```python
from build123d import *

# Parameters (mm, degrees)
SKETCH_1_W          = 92
SKETCH_1_H          = 30
SKETCH_1_R          = 1.05
EXTRUDE_1_DEPTH     = 4
SKETCH_4_W          = 92
SKETCH_4_H          = 30
EXTRUDE_4_DEPTH     = 4
SKETCH_5_W          = 92
SKETCH_5_H          = 34
SKETCH_5_R          = 1.05
EXTRUDE_5_DEPTH     = 4
FILLET_4_R          = 2
CUT_EXTRUDE_1_DEPTH = 45
SKETCH_8_R          = 2.55
CUT_EXTRUDE_2_DEPTH = 5
SKETCH_9_W          = 7
SKETCH_9_H          = 21
SKETCH_9_R          = 1.05
EXTRUDE_6_DEPTH     = 6


with BuildPart() as part:
    # 草图1 → 凸台-拉伸1 (new body)
    with BuildSketch(Plane.XY):
        with Locations((46, -15)):
            Rectangle(SKETCH_1_W, SKETCH_1_H)
        with Locations((3.5, -5)):
            Circle(SKETCH_1_R, mode=Mode.SUBTRACT)
        with Locations((3.5, -20)):
            Circle(SKETCH_1_R, mode=Mode.SUBTRACT)
        with Locations((88.5, -5)):
            Circle(SKETCH_1_R, mode=Mode.SUBTRACT)
        with Locations((88.5, -20)):
            Circle(SKETCH_1_R, mode=Mode.SUBTRACT)
        with BuildLine():
            Line((43.45, -17.5), (43.45, -7.5))
            ThreePointArc((43.45, -7.5), (46, -4.95), (48.55, -7.5))
            Line((48.55, -7.5), (48.55, -17.5))
            ThreePointArc((48.55, -17.5), (46, -20.05), (43.45, -17.5))
        make_face(mode=Mode.SUBTRACT)
    extrude(amount=EXTRUDE_1_DEPTH)

    # 草图4 → 凸台-拉伸4 (add)
    with BuildSketch(Plane(origin=(0, -30, 0), x_dir=(-1, 0, 0), z_dir=(0, -1, 0))):
        with Locations((-46, -15)):
            Rectangle(SKETCH_4_W, SKETCH_4_H)
    extrude(amount=EXTRUDE_4_DEPTH)

    # 草图5 → 凸台-拉伸5 (add)
    with BuildSketch(Plane.XY.offset(30)):
        with Locations((46, -17)):
            Rectangle(SKETCH_5_W, SKETCH_5_H)
        with Locations((3.5, -5)):
            Circle(SKETCH_5_R, mode=Mode.SUBTRACT)
        with Locations((3.5, -20)):
            Circle(SKETCH_5_R, mode=Mode.SUBTRACT)
        with Locations((88.5, -20)):
            Circle(SKETCH_5_R, mode=Mode.SUBTRACT)
        with Locations((88.5, -5)):
            Circle(SKETCH_5_R, mode=Mode.SUBTRACT)
    extrude(amount=EXTRUDE_5_DEPTH)

    # 圆角4
    fillet_4_edges = [part.edges().sort_by_distance(p)[0] for p in [
        (46, -30, 30),
        (46, -34, 0),
        (46, -34, 34),
        (0, 0, 32),
        (92, 0, 32),
        (0, 0, 2),
        (92, 0, 2),
        (46, -30, 4),
    ]]
    fillet(fillet_4_edges, radius=FILLET_4_R)

    # 草图7 → 切除-拉伸1 (cut)
    with BuildSketch(Plane(origin=(0, 0, 0), x_dir=(-1, 0, 0), z_dir=(0, 0, -1))):
        with BuildLine():
            Line((-48.55, -17.5), (-48.55, -7.5))
            ThreePointArc((-48.55, -7.5), (-46, -4.95), (-43.45, -7.5))
            Line((-43.45, -7.5), (-43.45, -17.5))
            ThreePointArc((-43.45, -17.5), (-46, -20.05), (-48.55, -17.5))
        make_face()
    extrude(amount=-CUT_EXTRUDE_1_DEPTH, mode=Mode.SUBTRACT)

    # 草图8 → 切除-拉伸2 (cut)
    with BuildSketch(Plane(origin=(0, -34, 0), x_dir=(-1, 0, 0), z_dir=(0, -1, 0))):
        with Locations(Location((-46, -16.5, 0), (0, 0, 90))):
            Circle(SKETCH_8_R)
    extrude(amount=-CUT_EXTRUDE_2_DEPTH, mode=Mode.SUBTRACT)

    # 草图9 → 凸台-拉伸6 (add)
    # profile 1 of 2: a face of its own
    with BuildSketch(Plane.XY.offset(4)):
        with Locations((88.5, -12.5)):
            Rectangle(SKETCH_9_W, SKETCH_9_H)
        with Locations((88.5, -5)):
            Circle(SKETCH_9_R, mode=Mode.SUBTRACT)
        with Locations((88.5, -20)):
            Circle(SKETCH_9_R, mode=Mode.SUBTRACT)
    # profile 2 of 2: a face of its own
    with BuildSketch(Plane.XY.offset(4)):
        with Locations((3.5, -12.5)):
            Rectangle(SKETCH_9_W, SKETCH_9_H)
        with Locations((3.5, -5)):
            Circle(SKETCH_9_R, mode=Mode.SUBTRACT)
        with Locations((3.5, -20)):
            Circle(SKETCH_9_R, mode=Mode.SUBTRACT)
    extrude(amount=EXTRUDE_6_DEPTH)


solid = part.part
```
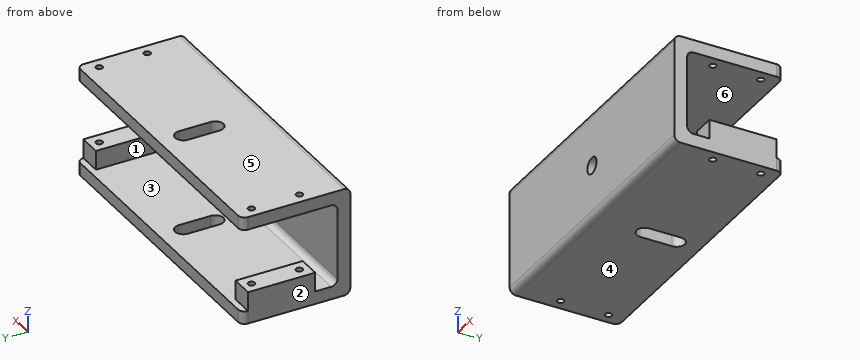
Work out the finished part from the listing and answer in its coordinate system (mm). Face numbers are marked on the shaded views. A direction names the side the tool comes from. Coordinates: 2 decimals unless noted, no trailing zeros. Write each loop counter-clockwise with the first axis right and the second up, starting at its lowest first coordinate (ties: lowest second). Pieces come first, ordered by that corner, then holes. Notation, with made-up numbers: (77.25, -2) - (128.25, -2) arc R27 cw to (128.25, 14) - close; hole circle Ø6 at (-29, 19.25). An arc over 180 degrees is marked (long way). Answer as a JSON object with one key per item and string values.
Q1. Find section D-D (x = 46). Write down the section's boundary in (y, z), plus the area to 3 significant figures.
Results list:
{"outline": "(-34, 2) arc R2 ccw to (-32, 0) - (-20.05, 0) - (-20.05, 4) - (-28, 4) arc R2 cw to (-30, 6) - (-30, 13.95) - (-34, 13.95) - close; (-34, 19.05) - (-30, 19.05) - (-30, 28) arc R2 cw to (-28, 30) - (-20.05, 30) - (-20.05, 34) - (-32, 34) arc R2 ccw to (-34, 32) - close; (-4.95, 0) - (0, 0) - (0, 4) - (-4.95, 4) - close; (-4.95, 30) - (0, 30) - (0, 34) - (-4.95, 34) - close", "area": "235 mm^2"}
Q2. Find section C-C (y = -26). Write down the section's boundary in (x, z), plus the area to 3 significant figures.
Results list:
{"outline": "(0, 0) - (92, 0) - (92, 4) - (0, 4) - close; (0, 30) - (92, 30) - (92, 34) - (0, 34) - close", "area": "736 mm^2"}
Q3. Consider L1, parallel to Y at x = 3.5, z = 2.5; L2, parallel to Z at x = 66, y = -12.5; L3, parallel to X at y = -2.5, z = 7.5. Determine where each line is inside the solid, lowest interval first. Write a range as from..to.
Results list:
{"L1": "y = -34..-21.05, -18.95..-6.05, -3.95..0", "L2": "z = 0..4, 30..34", "L3": "x = 0..7, 85..92"}
Q4. Find section B-B (z = 16.5). Write down the section's boundary in (x, y).
Results list:
{"outline": "(0, -34) - (43.45, -34) - (43.45, -30) - (0, -30) - close; (48.55, -34) - (92, -34) - (92, -30) - (48.55, -30) - close"}
Q5. Given pin 1 Ø1.3 at (x, y) = (88.5, -20) entering from +Z; pin 2 Ø6.5 at (x, z) = (4, 7.5) entering from +Y, each flat-ended and moving along its own axis, determine where each tip first touches the part or whether it passes through.
Results list:
{"pin 1": "passes through", "pin 2": "stops at y = -2"}
Q6. Which of the six approach directions +Z, -Z, +X, -X, +Y, -Y give full straight-line access (tool end or side, diameter ignored) to the marked faces 1 and 2?
Results list:
{"face 1": "+Y", "face 2": "+Z, -Z, -X, +Y, -Y"}
Q7. For a pull along Z with two mould halves and no side action, classify the marked faces 3, 4, 5 and 6 as pulls with the +Z half, pulls with the -Z half, needs draft (parallel to the pull), parting line crosses it, or undercut.
Results list:
{"face 3": "undercut", "face 4": "pulls with the -Z half", "face 5": "pulls with the +Z half", "face 6": "undercut"}
Q8. Find section A-A (x = 3.5). State how many separate pieces and enclosed holes the cut face has, plus the area to 3 significant figures.
Results list:
{"separate pieces": "5", "enclosed holes": "0", "area": "443 mm^2"}
